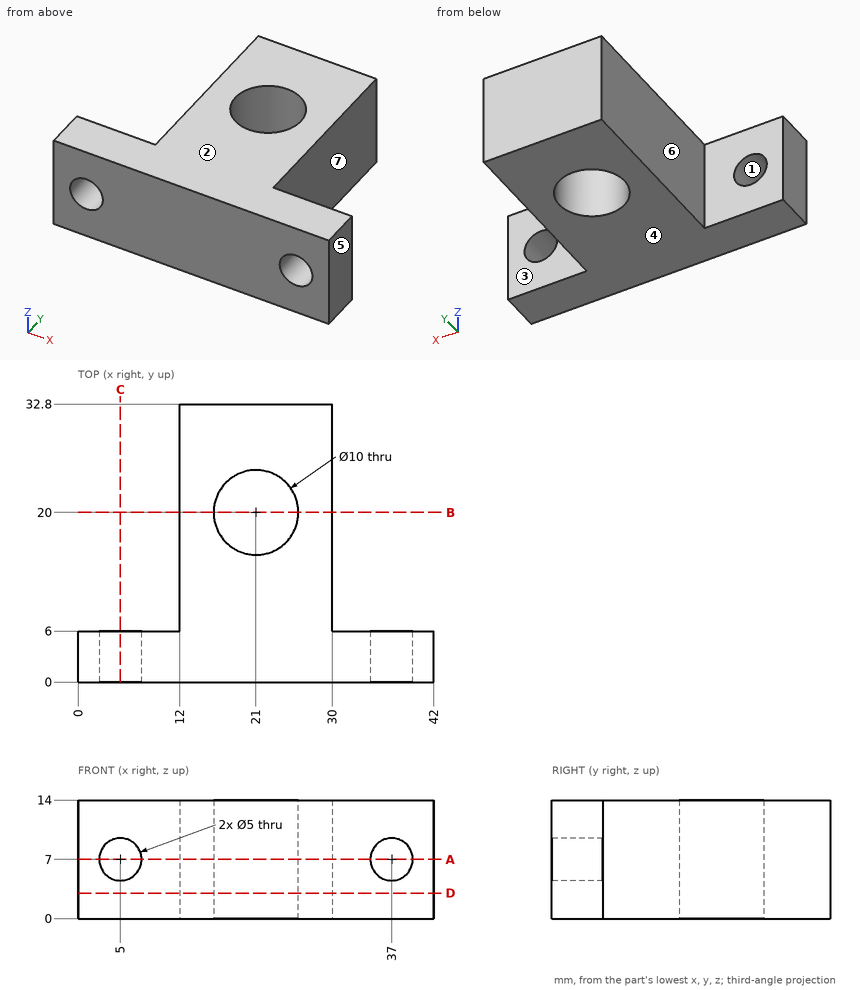
Check sheet for the drawn part. Datum: minimum x, y, z corner. Units: mm. A direction names the side the tool comes from. Coordinates: 2 decimals unless noted, no trailing zeros. Order: outer loops, then holes, each group sorted by start corner. A loop starts at its lowest first (then second) coordinate and runs counter-clockwise, first axis right, second up. Notation, with made-up numbers: (-8, 75) -> (12, 75) arc R20 cw to (12, 91) -> close; hole circle Ø2 at (26, 8). An arc over 180 degrees is marked (long way). Write each question's results on one line, items separated by ' | '. Start each with the question number.
1) Set-up check for the marked faces 5, 6 and 7: record each of +Z, -Z, +X, -X, +Y, -Y from which the full face is reachable in a straight line by a thin tool's end or side.
2) Section check C-C (x = 5). Enter the section's corners in (y, z).
3) Draft check along Z on the marked faces 1, 2, 3 and 4. Enter one of: pulls with the +Z half, pulls with the -Z half, needs draft (parallel to the pull), parting line crosses it, or undercut.
4) Material ranges on line 1 along Y through (x, z) = (21, 5.5); line 2 along Y through (x, z) = (9.5, 2); line 3 along X through (y, z) = (11.5, 6), recorded low to high.
5) Depth check by flat-ended pin: pin 1 (4 mm diameter, centred on y = 23.5, z = 5, fed in from -X); pin 2 (3.5 mm diameter, centred on x = 37, z = 8.5, fed in from +Y); pin 3 (8 mm diameter, centred on y = 24, z = 5.5, fed in from +X). Enter the tip coordinate at first touch or a pass-through.
6) Section check B-B (y = 20). Enter the section's corners in (x, z), and give its area (3 significant figures).
7) Section check A-A (z = 7). Enter the section's corners in (x, y).
8) Section check D-D (z = 3). Enter the section's corners in (x, y).
Checked values:
1) face 5: +Z, -Z, +X, +Y, -Y | face 6: +Z, -Z, -X, +Y | face 7: +Z, -Z, +X, +Y
2) outline: (0, 0) -> (6, 0) -> (6, 4.5) -> (0, 4.5) -> close; (0, 9.5) -> (6, 9.5) -> (6, 14) -> (0, 14) -> close
3) face 1: undercut | face 2: pulls with the +Z half | face 3: needs draft | face 4: pulls with the -Z half
4) line 1: 0 to 15, 25 to 32.8 | line 2: 0 to 6 | line 3: 12 to 30
5) pin 1: x = 12 | pin 2: y = 6 | pin 3: x = 30
6) outline: (12, 0) -> (16, 0) -> (16, 14) -> (12, 14) -> close; (26, 0) -> (30, 0) -> (30, 14) -> (26, 14) -> close | area: 112 mm²
7) outline: (0, 0) -> (2.5, 0) -> (2.5, 6) -> (0, 6) -> close; (7.5, 0) -> (34.5, 0) -> (34.5, 6) -> (30, 6) -> (30, 32.8) -> (12, 32.8) -> (12, 6) -> (7.5, 6) -> close; (39.5, 0) -> (42, 0) -> (42, 6) -> (39.5, 6) -> close; hole circle Ø10 at (21, 20)
8) outline: (0, 0) -> (42, 0) -> (42, 6) -> (30, 6) -> (30, 32.8) -> (12, 32.8) -> (12, 6) -> (0, 6) -> close; hole circle Ø10 at (21, 20)
